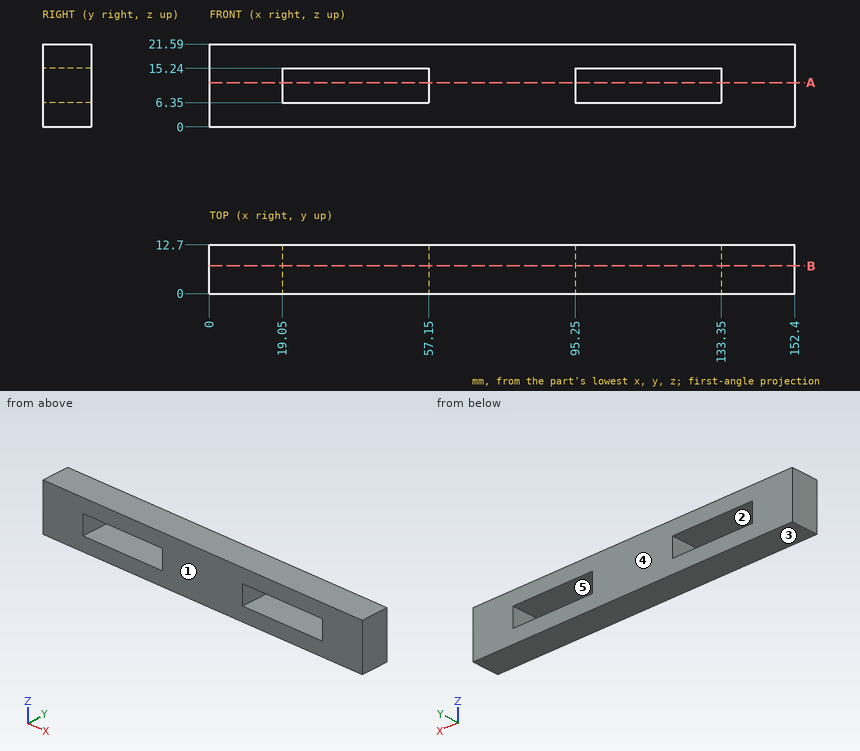
Check sheet for the drawn part. Datum: minimum x, y, z corner. Units: mm. A direction names the side the tool comes from. Give positions to 0.01 mm unless a question says otherwise; leave off trailing zeros. Order: outer loops, then holes, each group sorted by start corner. A loop starts at its lowest first (then second) coordinate and runs counter-clockwise, first axis right, second up. Notation, with made-up numbers: (39.25, 7) -> (92.25, 7) arc R20 ccw to (92.25, 44) -> close; hole circle Ø7 at (38.25, 9). An arc over 180 degrees is marked (long way). Return JSON: item names as keys, results as strings.
1. Cross-section at A-A, the plane z = 11.5. Record the cut outline in (x, y), plus the area to 3 significant figures.
From the geometry:
{"outline": "(0, 0) -> (19.05, 0) -> (19.05, 12.7) -> (0, 12.7) -> close; (57.15, 0) -> (95.25, 0) -> (95.25, 12.7) -> (57.15, 12.7) -> close; (133.35, 0) -> (152.4, 0) -> (152.4, 12.7) -> (133.35, 12.7) -> close", "area": "968 mm^2"}
2. Set-up check for the marked faces 1 and 2: record each of +Z, -Z, +X, -X, +Y, -Y from which the full face is reachable in a straight line by a thin tool's end or side.
From the geometry:
{"face 1": "+Z, -Z, +X, -X, -Y", "face 2": "+Y, -Y"}
3. Mould release check, pull along Z, two halves, no side actions. Record for the marked faces 3, 4 and 5: +Z half, -Z half, draft (parallel to the pull), parting line (faces both ways), or undercut.
From the geometry:
{"face 3": "-Z half", "face 4": "draft", "face 5": "undercut"}
4. Material ranges on probe 1 along X at (y, z) = (11.25, 13); probe 2 along Z at (x, y) = (97.5, 8), recorded low to high. Write a range as [from, to].
From the geometry:
{"probe 1": "[0, 19.05], [57.15, 95.25], [133.35, 152.4]", "probe 2": "[0, 6.35], [15.24, 21.59]"}
5. Cross-section at B-B, the plane y = 7.25. Record the cut outline in (x, z), plus the area to 3 significant figures.
From the geometry:
{"outline": "(0, 0) -> (152.4, 0) -> (152.4, 21.59) -> (0, 21.59) -> close; hole (19.05, 6.35) -> (57.15, 6.35) -> (57.15, 15.24) -> (19.05, 15.24) -> close; hole (95.25, 6.35) -> (133.35, 6.35) -> (133.35, 15.24) -> (95.25, 15.24) -> close", "area": "2,610 mm^2"}
